```python
from build123d import *

# Parameters (mm, degrees)
SKETCH1_R           = 1.6
SKETCH1_R_2         = 3
SKETCH1_R_3         = 7.6
SKETCH1_W           = 9
SKETCH1_H           = 9
BOSS_EXTRUDE1_DEPTH = 3.175
FILLET1_R           = 10
MIRROR2_OUTLINE_R   = 3
MIRROR2_OUTLINE_R_2 = 1.6
MIRROR2_DEPTH       = 3.175


# Read off the part's stored shape, not the designer's step: Mirror2
with BuildPart() as part:
    # Sketch1 → Boss-Extrude1 (new body)
    # profile 1 of 2: a face of its own
    with BuildSketch(Plane(origin=(0, 0, 0), x_dir=(1, 0, 0), z_dir=(0, 1, 0))):
        with BuildLine():
            ThreePointArc((23.66850222, -9.217483532), (0, -25.4), (-23.66850222, -9.217483532))
            Line((-23.66850222, -9.217483532), (-65.553741095, 98.334742178))
            Line((-65.553741095, 98.334742178), (-35.96811332, 109.856596592))
            Line((-35.96811332, 109.856596592), (0, 17.498268312))
            Line((0, 17.498268312), (35.96811332, 109.856596592))
            Line((35.96811332, 109.856596592), (65.553741095, 98.334742178))
            Line((65.553741095, 98.334742178), (23.66850222, -9.217483532))
        make_face()
        with Locations(Location((-15.161153788, 5.181560445, 0), (0, 0, 270))):
            Circle(SKETCH1_R, mode=Mode.SUBTRACT)
        with Locations(Location((-20.686165487, 26.870192161, 0), (0, 0, 270))):
            Circle(SKETCH1_R_2, mode=Mode.SUBTRACT)
        with Locations(Location((-45, 89.302855497, 0), (0, 0, 270))):
            Circle(SKETCH1_R_3, mode=Mode.SUBTRACT)
        with Locations(Location((45, 89.302855497, 0), (0, 0, 270))):
            Circle(SKETCH1_R_3, mode=Mode.SUBTRACT)
        Rectangle(SKETCH1_W, SKETCH1_H, mode=Mode.SUBTRACT)
    # profile 2 of 2: a face of its own
    with BuildSketch(Plane(origin=(0, 0, 0), x_dir=(1, 0, 0), z_dir=(0, 1, 0))):
        with BuildLine():
            Line((-23.66850222, -9.217483532), (-34.882073701, 19.576540408))
            ThreePointArc((-34.882073701, 19.576540408), (0, -40), (34.882073701, 19.576540408))
            Line((34.882073701, 19.576540408), (23.66850222, -9.217483532))
            ThreePointArc((23.66850222, -9.217483532), (0, -25.4), (-23.66850222, -9.217483532))
        make_face()
        with Locations(Location((-32.458777971, 7.835274371, 0), (0, 0, 270))):
            Circle(SKETCH1_R, mode=Mode.SUBTRACT)
    extrude(amount=BOSS_EXTRUDE1_DEPTH)

    # Fillet1
    fillet1_edges = [part.edges().sort_by_distance(p)[0] for p in [
        (-65.553741095, 1.5875, -98.334742178),
        (-35.96811332, 1.5875, -109.856596592),
        (35.96811332, 1.5875, -109.856596592),
        (65.553741095, 1.5875, -98.334742178),
    ]]
    fillet(fillet1_edges, radius=FILLET1_R)

    # Mirror2 outline → Mirror2 (cut)
    with BuildSketch(Plane(origin=(0, 0, 0), x_dir=(1, 0, 0), z_dir=(0, 1, 0))):
        with Locations((20.686165487, 26.870192161)):
            Circle(MIRROR2_OUTLINE_R)
        with Locations((15.161153788, 5.181560445)):
            Circle(MIRROR2_OUTLINE_R_2)
        with Locations((32.458777971, 7.835274371)):
            Circle(MIRROR2_OUTLINE_R_2)
    extrude(amount=MIRROR2_DEPTH, mode=Mode.SUBTRACT)


solid = part.part
```
CAD build for the part. Positions are in the model's coordinates, mm. A direction names the side the tool comes from. Round coordinates to 2 decimals unless told otherwise and drop trailing zeros. Order: outer loops, then holes, each group sorted by start corner. A loop starts at its lowest first (then second) coordinate and runs counter-clockwise, first axis right, second up.
Item 1: Probe line 1 along X through (y, z) = (1.8, -86.5); line 2 along X through (y, z) = (2.45, -6); line 3 along X through (y, z) = (0.95, 0.5). List the from-to ranges inside material, lowest first.
Item 2: Pin check, flat tips, straight feed: pin 1 (2.5 mm diameter, centred on x = 32.46, z = -7.84, fed in from +Y); pin 2 (1.6 mm diameter, centred on x = -1.5, y = 2, fed in from +Z); pin 3 (1 mm diameter, centred on y = 2, z = 2, fed in from -X); pin 4 (1 mm diameter, centred on y = 1.5, z = -32, fed in from -X) (3 decimals). Stop position of each tip, or through.
Item 3: Tool access for faces 4 (the face through (-48.214, 1.565, -53.81)), 5 (the face through (15.943, 1.565, -58.437)), 6 (the face through (-4.5, 2, 0)): list every direction of +Z, -Z, +X, -X, +Y, -Y with a clear straight run to the whole face (end or side of a thin tool).
Item 4: Mould opens along X. For faces 1 (the face through (-61.805, 1.61, -96.567)), 2 (the face through (50.684, 1.565, -104.126)), 3 (the face through (0, 2, -4.5)) say: pulls with the +X half, pulls with the -X half, needs draft (parallel to the pull), parting line crosses it, or undercut.
Item 5: Saw through at B-B on y = 2.3. State how many separate pieces and enclosed holes the cut face has, then the cut area to 3 significant figures.
Item 6: Saw through at D-D on z = 23. Write the cut outline in (x, y) (3 decimals).
Item 7: Saw through at C-C on z = -69. Write the cut outline in (x, y) (3 decimals).
Item 8: Saw through at A-A on z = 0. Write the cut outline in (x, y) (3 decimals).
Reported:
1. line 1: x = -60.94 to -52.06, -37.94 to -26.87, 26.87 to 37.94, 52.06 to 60.94
1. line 2: x = -39.55 to -16.54, -13.79 to 13.79, 16.54 to 39.55
1. line 3: x = -40 to -4.5, 4.5 to 40
2. pin 1: passes through
2. pin 2: stops at z = 39.99
2. pin 3: stops at x = -39.97
2. pin 4: stops at x = -39.915
3. face 4: -X, +Y, -Y
3. face 5: -Z, +Y, -Y
3. face 6: +Y, -Y
4. face 1: pulls with the -X half
4. face 2: pulls with the +X half
4. face 3: undercut
5. separate pieces: 1
5. enclosed holes: 9
5. area: 9,150 mm2
6. outline: (-32.726, 0) - (32.726, 0) - (32.726, 3.175) - (-32.726, 3.175) - close
7. outline: (-54.13, 0) - (-20.057, 0) - (-20.057, 3.175) - (-54.13, 3.175) - close; (20.057, 0) - (54.13, 0) - (54.13, 3.175) - (20.057, 3.175) - close
8. outline: (-40, 0) - (-4.5, 0) - (-4.5, 3.175) - (-40, 3.175) - close; (4.5, 0) - (40, 0) - (40, 3.175) - (4.5, 3.175) - close
